Autodesk Inventor part; units mm, degrees
ref_plane "YZ Plane" through (0, 0, 0) normal (1, 0, 0) x (0, 1, 0)
ref_plane "XZ Plane" through (0, 0, 0) normal (0, 1, 0) x (-1, 0, 0)
ref_plane "XY Plane" through (0, 0, 0) normal (0, 0, 1) x (1, 0, 0)
sketch "Sketch1" plane through (0, 0, 0) normal (0, 1, 0) x (-1, 0, 0)
  line L0 (25.4, 152.4) -> (-25.4, 152.4)
  line L1 (-25.4, 152.4) -> (-25.4, -152.4)
  line L2 (-25.4, -152.4) -> (25.4, -152.4)
  line L3 (25.4, -152.4) -> (25.4, 152.4)
  point P0 (0, 0)
  dimension "d0" = 50.8
  dimension "d1" = 304.8
  dimension "d2" = 152.4
  dimension "d3" = 25.4
extrude "Extrusion1" add sketch "Sketch1" along normal blind 6.35
sketch "Sketch2" plane through (0, 0, 0) normal (0, -1, 0) x (1, 0, 0)
  line L0 (-25.4, -152.4) -> (-25.4, 152.4)
  line L1 (-25.4, 152.4) -> (-19.05, 152.4)
  line L2 (-19.05, 152.4) -> (-19.05, -153.9502)
  line L3 (-19.05, -153.9502) -> (-25.4, -153.9502)
  line L4 (-25.4, -153.9502) -> (-25.4, 152.4)
  point P0 (0, 0)
  dimension "d6" = 6.35
extrude "Extrusion2" add sketch "Sketch2" against normal blind 50.8
sketch "Sketch3" plane through (-25.4, 0, -153.9502) normal (-1, 0, 0) x (0, 0, 1)
  line L0 (153.9502, 0) -> (153.1751, 50.8) construction
  line L1 (0, 50.8) -> (306.3502, 50.8) construction
  line L2 (0, 0) -> (0, 50.8) construction
  line L3 (0, 25.4) -> (306.3502, 25.4) construction
  line L4 (306.3502, 0) -> (306.3502, 50.8) construction
  circle A0 centre (165.8751, 25.4) radius 4.7625
  circle A1 centre (254.7751, 25.4) radius 4.7625
  circle A2 centre (140.4751, 25.4) radius 4.7625
  circle A3 centre (51.5751, 25.4) radius 4.7625
  point P0 (153.1751, 25.4)
  dimension "d9" = 9.525
  dimension "d10" = 12.7
  dimension "d11" = 12.7
  dimension "d12" = 101.6
  dimension "d13" = 88.9
extrude "Extrusion3" cut sketch "Sketch3" against normal blind 50.8
properties part number "L-Bracket"
Can you work these out from the model? Positions are in its coordinate system, mm. Round coordinates to 2 decimals unless told otherwise and drop trailing zeros. Order: outer loops, then holes, each group sorted by start corner. A loop starts at its lowest first (then second) coordinate and runs counter-clockwise, first axis right, second up. Notation, with made-up numbers: (-15.5, 47.25) -> (26.5, 47.25) arc R15 cw to (26.5, 51.25) -> close; hole circle Ø3 at (62, 86). An arc over 180 degrees is marked (long way). Return JSON: item names as keys, results as strings. Group by question number.
1. If we section it at B-B, the plane z = -104: Write out the boundary of the cut face in (x, y).
2. I need wall thicknesses on line 1 (Z direction, x = -20, y = 25); line 2 (X direction, y = 27, z = 19); line 3 (Y direction, x = 23, z = 27). Which ranges of each line are inside material? Lowest first, please. Write a range as [from, to].
3. If we section it at A-A, the plane y = 25.4: Write out the boundary of the cut face in (x, z), then the cut area to 3 significant figures.
4. If we section it at C-C, the plane x = 14: Write out the boundary of the cut face in (y, z).
5. Will these pins go through, and if not, where does the flat tip stop? pin 1 (12.5 mm diameter, centred on y = 25.4, z = -102.38, fed in from +X); pin 2 (7 mm diameter, centred on x = -5, y = 1.5, fed in from -Z); pin 3 (2 mm diameter, centred on x = -17, z = -24.5, fed in from +Y); pin 4 (12.5 mm diameter, centred on y = 25.4, z = -13.48, fed in from -X).
6. We'd pull the mould along Y, two halves only. Please class faces 1 (the face through (3, 3, -152.4)), 2 (the face through (3, 6.35, 2)), 3 (the face through (-22.269, 29.416, -10.915)): released by +Y, released by -Y, zero draft, split by the parting line, or undercut.
Output values:
{
 "1": {"outline": "(-25.4, 0) -> (25.4, 0) -> (25.4, 6.35) -> (-19.05, 6.35) -> (-19.05, 20.92) -> (-25.4, 20.92) -> close; (-25.4, 29.88) -> (-19.05, 29.88) -> (-19.05, 50.8) -> (-25.4, 50.8) -> close"},
 "2": {"line 1": "[-153.95, -107.12], [-97.63, -18.22], [-8.73, 7.18], [16.67, 96.08], [105.57, 152.4]", "line 2": "[-25.4, -19.05]", "line 3": "[0, 6.35]"},
 "3": {"outline": "(-25.4, -153.95) -> (-19.05, -153.95) -> (-19.05, -107.14) -> (-25.4, -107.14) -> close; (-25.4, -97.61) -> (-19.05, -97.61) -> (-19.05, -18.24) -> (-25.4, -18.24) -> close; (-25.4, -8.71) -> (-19.05, -8.71) -> (-19.05, 7.16) -> (-25.4, 7.16) -> close; (-25.4, 16.69) -> (-19.05, 16.69) -> (-19.05, 96.06) -> (-25.4, 96.06) -> close; (-25.4, 105.59) -> (-19.05, 105.59) -> (-19.05, 152.4) -> (-25.4, 152.4) -> close", "area": "1,700 mm²"},
 "4": {"outline": "(0, -152.4) -> (6.35, -152.4) -> (6.35, 152.4) -> (0, 152.4) -> close"},
 "5": {"pin 1": "x = -19.05", "pin 2": "z = -152.4", "pin 3": "y = 6.35", "pin 4": "x = -25.4"},
 "6": {"face 1": "zero draft", "face 2": "released by +Y", "face 3": "undercut"}
}
